For this review, take the finished solid that the model builds, in its own axes (mm). Face numbers are marked on the shaded views. Round coordinates to 2 decimals unless told otherwise and drop trailing zeros. Order: outer loops, then holes, each group sorted by start corner. A loop starts at its lowest first (then second) coordinate and runs counter-clockwise, first axis right, second up. Notation, with made-up numbers: M 89,32.5 L 128,32.5 A23 cw 128,57.5 Z; hole C 39,65.5 d1. An arc over 180 degrees is marked long. Answer as a JSON object with one key per item and string values.
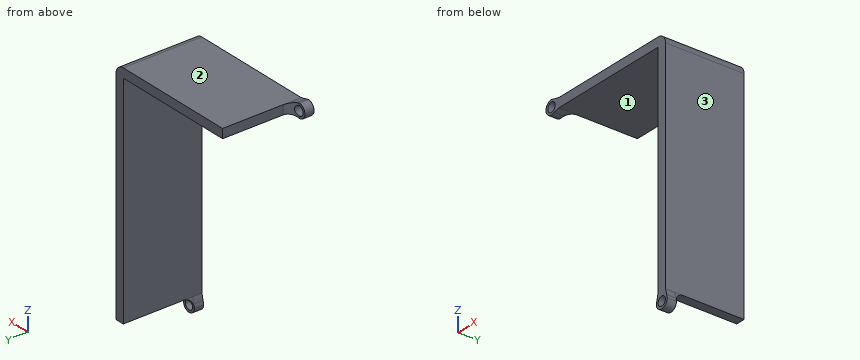
from build123d import *

# Parameters (mm, degrees)
SKETCH2_W           = 27
SKETCH2_H           = 17.15
BOSS_EXTRUDE1_DEPTH = 2
SKETCH3_W           = 48
SKETCH3_H           = 17.15
SKETCH3_W_2         = 2
BOSS_EXTRUDE2_DEPTH = 2
FILLET1_R           = 2
SKETCH4_R           = 1
BOSS_EXTRUDE3_DEPTH = 2
FILLET2_R           = 2


with BuildPart() as part:
    # Sketch2 → Boss-Extrude1 (new body)
    with BuildSketch(Plane.XY):
        with Locations((-0.118075802, 0.075)):
            Rectangle(SKETCH2_W, SKETCH2_H)
    extrude(amount=BOSS_EXTRUDE1_DEPTH)

    # Sketch3 → Boss-Extrude2 (add)
    with BuildSketch(Plane(origin=(13.381924198, 0, 0), x_dir=(0, 0, -1), z_dir=(1, 0, 0))):
        with Locations((24, 0.075)):
            Rectangle(SKETCH3_W, SKETCH3_H)
        with Locations((-1, 0.075)):
            Rectangle(SKETCH3_W_2, SKETCH3_H)
    extrude(amount=BOSS_EXTRUDE2_DEPTH)

    # Fillet1
    fillet1_edges = [part.edges().sort_by_distance(p)[0] for p in [
        (15.381924198, 0.075, 2),
    ]]
    fillet(fillet1_edges, radius=FILLET1_R)

    # Sketch4 → Boss-Extrude3 (add)
    # profile 1 of 4: a face of its own
    with BuildSketch(Plane.XZ.offset(8.5)):
        with BuildLine():
            Line((13.381924198, -48), (13.058394786, -49.294117647))
            ThreePointArc((13.058394786, -49.294117647), (14.381924198, -48.5), (15.70545361, -49.294117647))
            Line((15.70545361, -49.294117647), (15.381924198, -48))
            Line((15.381924198, -48), (13.381924198, -48))
        make_face()
    # profile 2 of 4: a face of its own
    with BuildSketch(Plane.XZ.offset(8.5)):
        with BuildLine():
            Line((13.058394786, -49.294117647), (12.881924198, -50))
            ThreePointArc((12.881924198, -50), (14.381924198, -51.5), (15.881924198, -50))
            Line((15.881924198, -50), (15.70545361, -49.294117647))
            ThreePointArc((15.70545361, -49.294117647), (14.381924198, -48.5), (13.058394786, -49.294117647))
        make_face()
        with Locations(Location((14.381924198, -50, 0), (0, 0, 270))):
            Circle(SKETCH4_R, mode=Mode.SUBTRACT)
    # profile 3 of 4: a face of its own
    with BuildSketch(Plane.XZ.offset(8.5)):
        with BuildLine():
            Line((-15.618075802, -0.5), (-14.912193449, -0.323529412))
            ThreePointArc((-14.912193449, -0.323529412), (-14.331836413, 0.228256367), (-14.118075802, 1))
            ThreePointArc((-14.118075802, 1), (-14.331836413, 1.771743633), (-14.912193449, 2.323529412))
            Line((-14.912193449, 2.323529412), (-15.618075802, 2.5))
            ThreePointArc((-15.618075802, 2.5), (-17.118075802, 1), (-15.618075802, -0.5))
        make_face()
        with Locations(Location((-15.618075802, 1, 0), (0, 0, 270))):
            Circle(SKETCH4_R, mode=Mode.SUBTRACT)
    # profile 4 of 4: a face of its own
    with BuildSketch(Plane.XZ.offset(8.5)):
        with BuildLine():
            Line((-14.912193449, -0.323529412), (-13.618075802, 0))
            Line((-13.618075802, 0), (-13.618075802, 2))
            Line((-13.618075802, 2), (-14.912193449, 2.323529412))
            ThreePointArc((-14.912193449, 2.323529412), (-14.331836413, 1.771743633), (-14.118075802, 1))
            ThreePointArc((-14.118075802, 1), (-14.331836413, 0.228256367), (-14.912193449, -0.323529412))
        make_face()
    extrude(amount=-BOSS_EXTRUDE3_DEPTH)

    # Fillet2
    # the kernel refuses this fillet: 2 mm, written as the material it adds along each edge
    with BuildSketch(Plane(origin=(-13.618075802, -6.5, -5), x_dir=(0, 1, 0), z_dir=(0, 0, 1))) as fillet2_piece_1_section:
        with BuildLine():
            CenterArc((FILLET2_R, FILLET2_R), FILLET2_R, 180, 90)
            Line((0, FILLET2_R), (0, 0))
            Line((0, 0), (FILLET2_R, 0))
        make_face()
    fillet2_piece_1 = extrude(amount=12, mode=Mode.PRIVATE)
    fillet2_piece_1 = split(fillet2_piece_1, bisect_by=Plane(origin=(-13.669858881, -6.170840666, 2.01294577), z_dir=(-0.24253562503633297, 0, -0.9701425001453319)), keep=Keep.TOP, mode=Mode.PRIVATE)
    fillet2_piece_1 = split(fillet2_piece_1, bisect_by=Plane(origin=(-14.177655248, -6.170840666, -0.139894862), z_dir=(-0.24253562503633314, 0, 0.9701425001453319)), keep=Keep.TOP, mode=Mode.PRIVATE)
    fillet2_piece_1 = fillet2_piece_1 - Plane(origin=(-15.618075802, -6.170840666, 1), x_dir=(0, 0, -1), z_dir=(0, -1, 0)) * Cylinder(1, 32, mode=Mode.PRIVATE)
    add(fillet2_piece_1)
    with BuildSketch(Plane(origin=(20.381924198, -6.5, -48), x_dir=(0, 1, 0), z_dir=(-1, 0, 0))) as fillet2_piece_2_section:
        with BuildLine():
            CenterArc((FILLET2_R, FILLET2_R), FILLET2_R, 180, 90)
            Line((0, FILLET2_R), (0, 0))
            Line((0, 0), (FILLET2_R, 0))
        make_face()
    fillet2_piece_2 = extrude(amount=12, mode=Mode.PRIVATE)
    fillet2_piece_2 = split(fillet2_piece_2, bisect_by=Plane(origin=(15.52181906, -6.170840666, -48.559579447), z_dir=(-0.9701425001453322, 0, -0.24253562503633172)), keep=Keep.TOP, mode=Mode.PRIVATE)
    fillet2_piece_2 = split(fillet2_piece_2, bisect_by=Plane(origin=(13.368978429, -6.170840666, -48.051783079), z_dir=(0.9701425001453319, 0, -0.24253562503633297)), keep=Keep.TOP, mode=Mode.PRIVATE)
    fillet2_piece_2 = fillet2_piece_2 - Plane(origin=(14.381924198, -6.170840666, -50), x_dir=(0, 0, -1), z_dir=(0, -1, 0)) * Cylinder(1, 32, mode=Mode.PRIVATE)
    add(fillet2_piece_2)


solid = part.part
1) Mouldability with a two-part tool opening along X and no side actions: class the marked faces 1, 2 and 3 as +X half, -X half, draft (parallel to the pull), parting line (faces both ways), or undercut.
Geometry check:
{"face 1": "undercut", "face 2": "draft", "face 3": "+X half"}
2) Add section B-B on y = -2. State the section outline as (x, z) points.
Geometry check:
{"outline": "M -13.62,0 L 13.38,0 L 13.38,-48 L 15.38,-48 L 15.38,0 A2 ccw 13.38,2 L -13.62,2 Z"}
3) Add section C-C on x = -13. State the section outline as (y, z) points, and give its area (3 significant figures).
Geometry check:
{"outline": "M -8.5,0 L 8.65,0 L 8.65,2 L -8.5,2 Z", "area": "34.3 mm²"}
4) Insertion check: P1, Ø2.5, axis at x = -15.62, z = 1, coming from the +Y side; P2, Ø5, axis at y = -0.5, z = -15, coming from the +X side; P3, Ø0.6, axis at y = -1, z = 1.5, coming from the -X side. Each pin has a flat end and moves straight along its axis. Give the tip position at first contact, or say it passes through.
Geometry check:
{"P1": "stops at y = -6.06", "P2": "stops at x = 15.38", "P3": "stops at x = -13.62"}
5) Add section D-D on z = -16. State the section outline as (x, y) points.
Geometry check:
{"outline": "M 13.38,-8.5 L 15.38,-8.5 L 15.38,8.65 L 13.38,8.65 Z"}
6) For L1, parallel to X at y = -7.95, z = -50; L2, parallel to X at y = 2.25, z = -15.5; L3, parallel to Z at x = 3.5, y = 2.5, list the stretches that pass through material, from the lowest coordinate up.
Geometry check:
{"L1": "x = 12.88 to 13.38, 15.38 to 15.88", "L2": "x = 13.38 to 15.38", "L3": "z = 0 to 2"}
7) Add section A-A on z = 1. State the section outline as (x, y) points.
Geometry check:
{"outline": "M -17.12,-8.5 L -16.62,-8.5 L -16.62,-6.5 L -17.12,-6.5 Z; M -14.62,-8.5 L 15.11,-8.5 L 15.11,8.65 L -13.62,8.65 L -13.62,-4.5 A2 cw -14.62,-6.23 Z"}
